Can you work these out from the model? Positions are in its coordinate system, mm. A direction names the side the tool comes from. Round coordinates to 2 decimals unless told otherwise and drop trailing zeros. Write each loop counter-clockwise with the first axis right and the second up, starting at its lowest first coordinate (ties: lowest second). Pieces come first, ordered by that corner, then holes. Notation, with made-up numbers: M 78.5,1 L 114.5,1 A24 cw 114.5,39 Z; hole C 89,80 d6. An arc over 180 degrees is marked long. Answer as a JSON object with one key per item and string values. Group by question number.
1) Suppose I cut it at B-B, the plane z = 14.5. Write out the boundary of the cut face in (x, y), and give its area (3 significant figures).
2) Suppose I cut it at C-C, the plane x = -7. Write out the boundary of the cut face in (y, z).
3) Suppose I cut it at D-D, the plane y = 2. Write out the boundary of the cut face in (x, z), and give its area (3 significant figures).
4) I'm going to push flat-ended pins straight in: pin 1 Ø1.5 at (x, y) = (-0.5, 14) entering from +Z; pin 2 Ø2.5 at (y, z) = (17.5, 12.5) entering from -X; pin 3 Ø2.5 at (x, y) = (-6.5, 13.5) entering from +Z; pin 4 Ø10 at (x, z) = (-5.5, 13.5) entering from -Y. Where does each tip first touch, or does it pass through?
5) Suppose I cut it at A-A, the plane y = 16.75. Write out the boundary of the cut face in (x, z).
6) On a 3-axis mill with a long thin cutter (end or side, diameter ignored), from which of +Z, -Z, +X, -X, +Y, -Y can I reach the whole of each face in a straight line? I mean faces 1 (the flat face through (-7, 15, 2)), 2 (the flat face through (1, 5, 17)), 3 (the flat face through (-3.536, 2, 14)). Say none if no direction works.
7) Please list where these lines run through material, in increasing order: L1, parallel to X at y = 16, z = 14.5; L2, parallel to Y at x = -6, z = 1; L3, parallel to X at y = 3.5, z = 15. Write a range as [from, to].
from build123d import *

# Parameters (mm, degrees)
BOSS_EXTRUDE1_DEPTH = 20
SKETCH3_W           = 5
SKETCH3_H           = 20
BOSS_EXTRUDE2_DEPTH = 5
CUT_EXTRUDE1_DEPTH  = 5
SKETCH5_W           = 5
SKETCH5_H           = 20
BOSS_EXTRUDE3_DEPTH = 5
CUT_EXTRUDE2_DEPTH  = 5
SKETCH7_W           = 5
SKETCH7_H           = 15
BOSS_EXTRUDE4_DEPTH = 5
BOSS_EXTRUDE6_DEPTH = 20
CUT_EXTRUDE4_DEPTH  = 31
BOSS_EXTRUDE7_DEPTH = 5


with BuildPart() as part:
    # Sketch2 → Boss-Extrude1 (new body)
    with BuildSketch(Plane(origin=(0, 0, 0), x_dir=(1, 0, 0), z_dir=(0, 1, 0))):
        Polygon((0, 0), (10, 0), (10, -15), (5, -15), (5, -10), (0, -5), align=None)
    extrude(amount=BOSS_EXTRUDE1_DEPTH)

    # Sketch3 → Boss-Extrude2 (add)
    with BuildSketch(Plane.XY.offset(15)):
        with Locations((7.5, 10)):
            Rectangle(SKETCH3_W, SKETCH3_H)
    extrude(amount=BOSS_EXTRUDE2_DEPTH)

    # Sketch4 → Cut-Extrude1 (cut)
    with BuildSketch(Plane.ZY.offset(-5)):
        Polygon((15, 20), (20, 15), (20, 20), align=None)
    extrude(amount=-CUT_EXTRUDE1_DEPTH, mode=Mode.SUBTRACT)

    # Sketch5 → Boss-Extrude3 (add)
    with BuildSketch(Plane.ZY):
        with Locations((2.5, 10)):
            Rectangle(SKETCH5_W, SKETCH5_H)
    extrude(amount=BOSS_EXTRUDE3_DEPTH)

    # Sketch6 → Cut-Extrude2 (cut)
    with BuildSketch(Plane.XY.offset(5)):
        Polygon((0, 20), (-5, 20), (-5, 15), align=None)
    extrude(amount=-CUT_EXTRUDE2_DEPTH, mode=Mode.SUBTRACT)

    # Sketch7 → Boss-Extrude4 (add)
    with BuildSketch(Plane.ZY.offset(5)):
        with Locations((2.5, 7.5)):
            Rectangle(SKETCH7_W, SKETCH7_H)
    extrude(amount=BOSS_EXTRUDE4_DEPTH)

    # Sketch8 → Boss-Extrude6 (add)
    with BuildSketch(Plane(origin=(0, 0, 0), x_dir=(-1, 0, 0), z_dir=(0, -1, 0))):
        Polygon((10, -5), (0, -5), (-5, -10), (-5, -15), (0, -15), align=None)
    extrude(amount=-BOSS_EXTRUDE6_DEPTH)

    # 3DSketch2 → Cut-Extrude4 (cut, along a direction that is not the sketch's normal)
    with BuildSketch(Plane(origin=(0, 20, 5), x_dir=(-0.7071067811865475, -0.7071067811865476, 0), z_dir=(-0.5773502691896257, 0.5773502691896257, 0.5773502691896257))):
        Polygon((0, 0), (-3.535533906, 6.123724357), (0, 12.247448714), (7.071067812, 12.247448714), (14.142135624, 0), align=None)
    extrude(amount=CUT_EXTRUDE4_DEPTH, dir=(0, 1, 0), mode=Mode.SUBTRACT)

    # Sketch9 → Boss-Extrude7 (add)
    with BuildSketch(Plane(origin=(0, 0, 0), x_dir=(-1, 0, 0), z_dir=(0, -1, 0))):
        Polygon((0, -15), (-5, -15), (-5, -20), (0, -20), (3.535533906, -16.464466094), (3.535533906, -11.464466094), align=None)
    extrude(amount=-BOSS_EXTRUDE7_DEPTH)


solid = part.part
Results:
{
 "1": {"outline": "M -3.54,0 L 10,0 L 10,20 L 5,20 L 5,15.5 L -0.5,10 L -0.5,5 L -3.54,5 Z", "area": "185 mm^2"},
 "2": {"outline": "M 0,0 L 15,0 L 15,5 L 13,5 L 10,8 L 0,8 Z"},
 "3": {"outline": "M -10,0 L 10,0 L 10,20 L 0,20 L -3.54,16.46 L -3.54,11.46 L -10,5 Z", "area": "318 mm^2"},
 "4": {"pin 1": "z = 11.56", "pin 2": "x = 3.23", "pin 3": "z = 6.77", "pin 4": "y = 0"},
 "5": {"outline": "M -3.25,0 L 10,0 L 10,18.25 L 5,18.25 L 5,13.25 L -3.25,5 Z"},
 "6": {"face 1": "+Z, -Z, -X, +Y", "face 2": "+Z, -X, +Y", "face 3": "+Z, -X, +Y, -Y"},
 "7": {"L1": "[5, 10]", "L2": "[0, 15]", "L3": "[-3.54, 10]"}
}
